```python
from build123d import *

# Parameters (mm, degrees)
F1_DEPTH = 23
F2_R     = 6.4008
F3_R     = 3.2004
F4_R     = 1.59766


with BuildPart() as f1:
    # F0 (on Top) → F1 (new body)
    with BuildSketch(Plane.XY):
        with BuildLine():
            Line((0, -50.775), (0, 0))
            Line((0, 0), (30, 0))
            Line((30, 0), (30, 3.2))
            Line((30, 3.2), (-3.2, 3.2))
            Line((-3.2, 3.2), (-3.2, -50.775))
            ThreePointArc((-3.2, -50.775), (-12.725, -60.3), (-22.25, -50.775))
            Line((-22.25, -50.775), (-25.45, -50.775))
            ThreePointArc((-25.45, -50.775), (-12.725, -63.5), (0, -50.775))
        make_face()
    extrude(amount=F1_DEPTH)

    # F2
    f2_edges = [f1.edges().sort_by_distance(p)[0] for p in [
        (-3.2, 3.2, 11.5),
    ]]
    fillet(f2_edges, radius=F2_R)

    # F3
    f3_edges = [f1.edges().sort_by_distance(p)[0] for p in [
        (0, 0, 11.5),
    ]]
    fillet(f3_edges, radius=F3_R)

    # F4
    f4_edges = [f1.edges().sort_by_distance(p)[0] for p in [
        (-25.45, -50.775, 11.5),
        (-22.25, -50.775, 11.5),
    ]]
    fillet(f4_edges, radius=F4_R)


solid = f1.part
```
For this review, take the finished solid that the model builds, in its own axes (mm). A direction names the side the tool comes from. Coordinates: 2 decimals unless noted, no trailing zeros. Loops run counter-clockwise (first coordinate to the right, second up) from the corner with the lowest first, then second, coordinate; pieces in that order, holes last.
1. Add section A-A, the plane y = -54. Give the boundary of the cut face in (x, z).
2. Add section B-B, the plane z = 8.5. Give the boundary of the cut face in (x, y) (3 decimals), then the cut area to 3 significant figures.
3. Insertion check: P1, Ø3, axis at y = -13.5, z = 13.5, coming from the +X side; P2, Ø5, axis at x = -7, z = 20.5, coming from the -Y side; P3, Ø1, axis at x = -14.5, z = 5.5, coming from the +Y side. Each pin has a flat end and moves straight along its axis. Give the tip position at first contact, or say it passes through.
4. Mouldability with a two-part tool opening along X and no side actions: class faces 1 (the cylindrical face through (-24.958, -51.342, 11.661)), 2 (the cylindrical face through (-22.699, -51.154, 11.661)), 3 (the cylindrical face through (-12.076, -63.483, 11.339)) as +X half, -X half, draft (parallel to the pull), parting line (faces both ways), or undercut.
5. For faces 4 (the flat face through (0, -27, 11)), 5 (the flat face through (-3.2, -27, 11)), 6 (the cylindrical face through (-11.84, -60.26, 11.34)), list the 3-axis set-ups (+Z, -Z, +X, -X, +Y, -Y) from which the entire face can be reached by the end or side of a thin tool; tool diameter is ignored.
6. For line 1 (Y direction, x = 26.5, z = 2.75); line 2 (X direction, y = -30, z = 6.75); line 3 (X direction, y = -55, z = 18), list the stretches that pass through material, from the lowest coordinate up.
7. Add section D-D, the plane x = -13.5. Give the boundary of the cut face in (y, z).
8. Add section C-C, the plane x = 6.5. Give the boundary of the cut face in (y, z), then the cut area to 3 significant figures.
Result:
1. outline: (-25.03, 0) - (-21.69, 0) - (-21.69, 23) - (-25.03, 23) - close; (-3.76, 0) - (-0.42, 0) - (-0.42, 23) - (-3.76, 23) - close
2. outline: (-25.318, -52.602) arc R12.725 ccw to (0, -50.775) - (0, -3.2) arc R3.2 cw to (3.2, 0) - (30, 0) - (30, 3.2) - (3.201, 3.2) arc R6.401 ccw to (-3.2, -3.201) - (-3.2, -50.775) arc R9.525 cw to (-22.151, -52.143) arc R1.598 ccw to (-23.732, -50.775) - (-23.737, -50.775) arc R1.598 ccw to start
2. area: 373 mm2
3. P1: stops at x = 0
3. P2: stops at y = -63.08
3. P3: stops at y = -60.02
4. face 1: -X half
4. face 2: undercut
4. face 3: parting line
5. face 4: +Z, -Z, +X, -Y
5. face 5: +Z, -Z, -X, +Y
5. face 6: +Z, -Z, +Y
6. line 1: y = 0 to 3.2
6. line 2: x = -3.2 to 0
6. line 3: x = -24.73 to -21.26, -4.19 to -0.72
7. outline: (-63.48, 0) - (-60.27, 0) - (-60.27, 23) - (-63.48, 23) - close
8. outline: (0, 0) - (3.2, 0) - (3.2, 23) - (0, 23) - close
8. area: 73.6 mm2
